```python
from build123d import *

# Parameters (mm, degrees)
CHAMFER1_SIZE           = 0.762
SKETCH5_W               = 6.35
SKETCH5_H               = 0.8001
CUT_EXTRUDE1_DEPTH      = 8.8613
CUT_EXTRUDE1_DEPTH_BACK = 8.8613
SKETCH6_W               = 6.35
SKETCH6_H               = 0.8001
CUT_EXTRUDE2_DEPTH      = 8.8613
CUT_EXTRUDE2_DEPTH_BACK = 8.8613


with BuildPart() as part:
    # Sketch1 → Revolve1 (revolve)
    with BuildSketch(Plane(origin=(0, 0, 0), x_dir=(-1, 0, 0), z_dir=(0, 0, -1)), mode=Mode.PRIVATE) as revolve1_sk:
        with BuildLine():
            Line((-76.708, 2.786922533), (-76.708, 0))
            Line((-76.708, 0), (0, 0))
            Line((0, 0), (0, 7.8613))
            Line((0, 7.8613), (-63.5, 7.8613))
            Line((-63.5, 7.8613), (-63.5, 3.175))
            Line((-63.5, 3.175), (-75.692, 3.175))
            ThreePointArc((-75.692, 3.175), (-76.235796865, 3.074678675), (-76.708, 2.786922533))
        make_face()
    revolve(revolve1_sk.sketch.rotate(Axis((76.708, 0, 0), (-1, 0, 0)), 270), axis=Axis((76.708, 0, 0), (-1, 0, 0)))  # turned: the seam where the file's is

    # Sketch2 → Cut-Revolve1 (revolve, cut)
    with BuildSketch(Plane(origin=(0, 0, 0), x_dir=(-1, 0, 0), z_dir=(0, 0, -1)), mode=Mode.PRIVATE) as cut_revolve1_sk:
        Polygon((-13.97, 4.9784), (-13.97, 0), (0, 0), (0, 6.1849), (-2.5527, 5.642306865), (-3.216606865, 4.9784), align=None)
    revolve(cut_revolve1_sk.sketch.rotate(Axis((13.97, 0, 0), (-1, 0, 0)), 270), axis=Axis((13.97, 0, 0), (-1, 0, 0)), mode=Mode.SUBTRACT)  # turned: the seam where the file's is

    # Sketch3 → Cut-Revolve2 (revolve, cut)
    with BuildSketch(Plane(origin=(0, 0, 0), x_dir=(-1, 0, 0), z_dir=(0, 0, -1)), mode=Mode.PRIVATE) as cut_revolve2_sk:
        Polygon((-76.708, 1.7272), (-76.708, 0), (-70.358, 0), (-71.395806461, 1.7272), align=None)
    revolve(cut_revolve2_sk.sketch.rotate(Axis((66.313858967, 0, 0), (-1, 0, 0)), 270), axis=Axis((66.313858967, 0, 0), (-1, 0, 0)), mode=Mode.SUBTRACT)  # turned: the seam where the file's is

    # Chamfer1
    chamfer1_edges = [part.edges().sort_by_distance(p)[0] for p in [
        (63.5, 0, -7.8613),
        (0, 0, -7.8613),
    ]]
    chamfer(chamfer1_edges, length=CHAMFER1_SIZE)

    # Sketch5 → Cut-Extrude1 (cut, two sides)
    with BuildSketch(Plane(origin=(0, 0, 0), x_dir=(1, 0, 0), z_dir=(0, 1, 0))) as cut_extrude1_sk:
        with Locations((3.175, 7.46125)):
            Rectangle(SKETCH5_W, SKETCH5_H)
        with Locations((3.175, -7.46125)):
            Rectangle(SKETCH5_W, SKETCH5_H)
    extrude(amount=CUT_EXTRUDE1_DEPTH, mode=Mode.SUBTRACT)
    extrude(cut_extrude1_sk.sketch, amount=-CUT_EXTRUDE1_DEPTH_BACK, mode=Mode.SUBTRACT)

    # Sketch6 → Cut-Extrude2 (cut, two sides)
    with BuildSketch(Plane(origin=(0, 0, 0), x_dir=(1, 0, 0), z_dir=(0, 1, 0))) as cut_extrude2_sk:
        with Locations((60.325, 7.46125)):
            Rectangle(SKETCH6_W, SKETCH6_H)
        with Locations((60.325, -7.46125)):
            Rectangle(SKETCH6_W, SKETCH6_H)
    extrude(amount=CUT_EXTRUDE2_DEPTH, mode=Mode.SUBTRACT)
    extrude(cut_extrude2_sk.sketch, amount=-CUT_EXTRUDE2_DEPTH_BACK, mode=Mode.SUBTRACT)


solid = part.part
```
Could you check a few things on this model? Use its own coordinates, in mm. A direction names the side the tool comes from. Round coordinates to 2 decimals unless told otherwise and drop trailing zeros. Order: outer loops, then holes, each group sorted by start corner. A loop starts at its lowest first (then second) coordinate and runs counter-clockwise, first axis right, second up. Notation, with made-up numbers: M 75,10 L 107,10 A22 ccw 107,34 Z; hole C 19.5,-11.75 d2. An arc over 180 degrees is marked long. One line per question, with ' | ' between items. Start each with the question number.
(1) For P1, Ø6, axis at y = 0.5, z = -3, coming from the +X side; P2, Ø3, axis at x = 25, z = 3.5, coming from the -Y side; P3, Ø1.9, axis at x = 4.5, y = 0, coming from the +Z side; P4, Ø8, axis at x = 16, y = -5.5, coming from the +Z side, each with a flat end and sliding along its axis, tell me the tip position at first contact or that it passes through.
(2) Suppose I cut it at A-A on x = 5. List the corners of the cut face in (y, z) for me.
(3) Thinking about a two-plate mould opening in Z: for faces 1 (the face through (0, -6, -3)), 2 (the face through (70.54, -0.27, 0.14)), 3 (the face through (69.68, -1.93, -2.52)), which applies, +Z half, -Z half, draft (parallel to the pull), parting line (faces both ways), or undercut?
(4) For faces 4 (the face through (63.5, -1.5, 3)), 5 (the face through (60, 0, 7.061)), 6 (the face through (8.669, 1.495, 4.749)), which set-ups out of +Z, -Z, +X, -X, +Y, -Y let a thin tool reach every point of the face, with its end or its side?
(5) Please list where these lines run through material, in increasing order: line 1 along Y through (x, z) = (74.8, 0) (3 decimals); line 2 along X through (y, z) = (-2, -4.5); line 3 along X through (y, z) = (-0.25, 6.75).
Geometry results:
1) P1: x = 76.71 | P2: y = -7.6 | P3: z = 7.06 | P4: z = 7.72
2) outline: M -3.46,-7.06 L 3.46,-7.06 A7.86 ccw 3.46,7.06 L -3.46,7.06 A7.86 ccw Z; hole C 0,0 d9.96
3) face 1: draft | face 2: undercut | face 3: parting line
4) face 4: +X | face 5: +Z, +X, +Y, -Y | face 6: -X
5) line 1: -3.175 to -1.727, 1.727 to 3.175 | line 2: 13.97 to 63.5 | line 3: 0 to 63.5
